Read the model definition and answer for the solid it produces. Units are mm, in the model's axes. Give positions to 0.01 mm unless a question says otherwise; leave off trailing zeros. Loops run counter-clockwise (first coordinate to the right, second up) from the corner with the lowest first, then second, coordinate; pieces in that order, holes last. Notation, with made-up numbers: (-35, 39) - (4, 39) arc R17 ccw to (4, 43) - close; hole circle Ø3 at (0, 14). An arc over 180 degrees is marked (long way). Write each question's results on one line, items separated by ' | '. Start each with the question number.
Q1. The part is cut by section B-B, the plane z = 0.5. Write down the section's boundary in (x, y).
Q2. Given pin 1 (3.5 mm diameter, centred on x = 12.5, y = -42.5, fed in from -Z), flat-ended and moving along its own axis, determine where the tip first touches the part or whether it passes through.
Q3. The part is cut by section D-D, the plane y = -22.5. Write down the section's boundary in (x, z), plus the area to 3 significant figures.
Q4. The part is cut by section A-A, the plane y = -42.5. Write down the section's boundary in (x, z), plus the area to 3 significant figures.
Q5. The part is cut by section C-C, the plane x = 42.5. Write down the section's boundary in (y, z).
Q6. Find the intervals of material crossed by line 1 (Y direction, x = 12.5, z = 0.7); line 2 (Y direction, x = 17, z = 0.5); line 3 (Y direction, x = 42.5, z = 2.2), in increasing order. Write a range as from..to.
```python
from build123d import *

# Parameters (mm, degrees)
SKETCH_1_R      = 1.5
SKETCH_1_W      = 15
SKETCH_1_H      = 15
EXTRUDE_1_DEPTH = 3
FILLET_1_R      = 5


with BuildPart() as part:
    # 草图1 → 凸台-拉伸1 (new body)
    with BuildSketch(Plane.XY):
        with BuildLine():
            Line((0, 0), (52.5, 0))
            Line((52.5, 0), (52.5, -20.5))
            ThreePointArc((52.5, -20.5), (47.122398776, -22.675796862), (43.857589438, -27.47097224))
            ThreePointArc((43.857589438, -27.47097224), (37.67766953, -37.67766953), (27.47097224, -43.857589438))
            ThreePointArc((27.47097224, -43.857589438), (22.675796862, -47.122398776), (20.5, -52.5))
            Line((20.5, -52.5), (0, -52.5))
            Line((0, -52.5), (0, 0))
        make_face()
        with Locations((22.5, -12.5)):
            Circle(SKETCH_1_R, mode=Mode.SUBTRACT)
        with Locations((42.5, -12.5)):
            Circle(SKETCH_1_R, mode=Mode.SUBTRACT)
        with Locations(Location((12.5, -42.5, 0), (0, 0, 180))):
            Circle(SKETCH_1_R, mode=Mode.SUBTRACT)
        with Locations(Location((12.5, -22.5, 0), (0, 0, 180))):
            Circle(SKETCH_1_R, mode=Mode.SUBTRACT)
        with Locations((27.5, -27.5)):
            Rectangle(SKETCH_1_W, SKETCH_1_H, mode=Mode.SUBTRACT)
    extrude(amount=EXTRUDE_1_DEPTH)

    # 圆角1
    fillet_1_edges = [part.edges().sort_by_distance(p)[0] for p in [
        (0, 0, 1.5),
        (52.5, 0, 1.5),
        (52.5, -20.5, 1.5),
        (20.5, -52.5, 1.5),
        (0, -52.5, 1.5),
    ]]
    fillet(fillet_1_edges, radius=FILLET_1_R)


solid = part.part
```
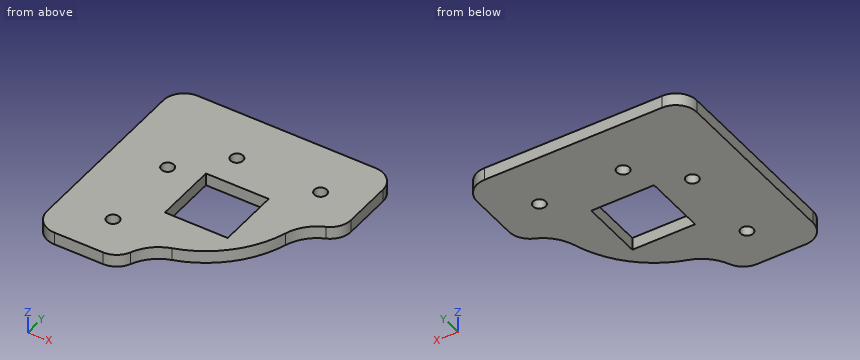
Check sheet entries:
1) outline: (0, -47.5) arc R5 ccw to (5, -52.5) - (16.67, -52.5) arc R5 ccw to (21.27, -49.47) arc R10 cw to (27.47, -43.86) arc R25 ccw to (43.86, -27.47) arc R10 cw to (49.47, -21.27) arc R5 ccw to (52.5, -16.67) - (52.5, -5) arc R5 ccw to (47.5, 0) - (5, 0) arc R5 ccw to (0, -5) - close; hole circle Ø3 at (12.5, -42.5); hole circle Ø3 at (12.5, -22.5); hole (20, -35) - (35, -35) - (35, -20) - (20, -20) - close; hole circle Ø3 at (22.5, -12.5); hole circle Ø3 at (42.5, -12.5)
2) pin 1: stops at z = 0
3) outline: (0, 0) - (11, 0) - (11, 3) - (0, 3) - close; (14, 0) - (20, 0) - (20, 3) - (14, 3) - close; (35, 0) - (47.35, 0) - (47.35, 3) - (35, 3) - close | area: 88.0 mm^2
4) outline: (0, 0) - (11, 0) - (11, 3) - (0, 3) - close; (14, 0) - (30.9, 0) - (30.9, 3) - (14, 3) - close | area: 83.7 mm^2
5) outline: (-30.9, 0) - (-14, 0) - (-14, 3) - (-30.9, 3) - close; (-11, 0) - (0, 0) - (0, 3) - (-11, 3) - close
6) line 1: y = -52.5..-44, -41..-24, -21..0 | line 2: y = -52.49..0 | line 3: y = -30.9..-14, -11..0
